Geometry: final body of the model. Coordinates: model frame, mm. A direction names the side the tool comes from. Coordinates: 2 decimals unless noted, no trailing zeros. Loops run counter-clockwise (first coordinate to the right, second up) from the corner with the lowest first, then second, coordinate; pieces in that order, holes last. Notation, with made-up numbers: (-11.75, 31) - (14.25, 31) arc R7 cw to (14.25, 36) - close; hole circle Ø11 at (-34.5, 88). An arc over 180 degrees is marked (long way). Answer in a Markdown table with one row per item.
from build123d import *

# Parameters (mm, degrees)
SKETCH1_W           = 76.2
SKETCH1_H           = 180.975
BOSS_EXTRUDE1_DEPTH = 5.08
SKETCH3_W           = 17.4625
SKETCH3_H           = 9.525
CUT_EXTRUDE1_DEPTH  = 6.08
SKETCH4_W           = 7.62
SKETCH4_H           = 4.826
CUT_EXTRUDE2_DEPTH  = 6.08


with BuildPart() as part:
    # Sketch1 → Boss-Extrude1 (new body)
    with BuildSketch(Plane.XY):
        Rectangle(SKETCH1_W, SKETCH1_H)
    extrude(amount=BOSS_EXTRUDE1_DEPTH)

    # Sketch3 → Cut-Extrude1 (cut, through all)
    with BuildSketch(Plane.XY.offset(5.08)):
        with Locations((0, -85.725)):
            Rectangle(SKETCH3_W, SKETCH3_H)
        with Locations((0, 85.725)):
            Rectangle(SKETCH3_W, SKETCH3_H)
    extrude(amount=-CUT_EXTRUDE1_DEPTH, mode=Mode.SUBTRACT)

    # Sketch4 → Cut-Extrude2 (cut, through all)
    with BuildSketch(Plane.XY.offset(5.08)):
        with Locations((-34.29, 40.513)):
            Rectangle(SKETCH4_W, SKETCH4_H)
        with Locations((34.29, 40.513)):
            Rectangle(SKETCH4_W, SKETCH4_H)
        with Locations((34.29, -40.513)):
            Rectangle(SKETCH4_W, SKETCH4_H)
        with Locations((-34.29, -40.513)):
            Rectangle(SKETCH4_W, SKETCH4_H)
    extrude(amount=-CUT_EXTRUDE2_DEPTH, mode=Mode.SUBTRACT)


solid = part.part
(1) Cut plane A-A on z = 0.8. Output: boundary loops of the cut face in (x, y), then the cut area to 3 significant figures.
Verdict:
| item | result |
|---|---|
| outline | (-38.1, -90.49) - (-8.73, -90.49) - (-8.73, -80.96) - (8.73, -80.96) - (8.73, -90.49) - (38.1, -90.49) - (38.1, -42.93) - (30.48, -42.93) - (30.48, -38.1) - (38.1, -38.1) - (38.1, 38.1) - (30.48, 38.1) - (30.48, 42.93) - (38.1, 42.93) - (38.1, 90.49) - (8.73, 90.49) - (8.73, 80.96) - (-8.73, 80.96) - (-8.73, 90.49) - (-38.1, 90.49) - (-38.1, 42.93) - (-30.48, 42.93) - (-30.48, 38.1) - (-38.1, 38.1) - (-38.1, -38.1) - (-30.48, -38.1) - (-30.48, -42.93) - (-38.1, -42.93) - close |
| area | 13,300 mm² |
(2) Pull-direction query (X, two-part tool) for faces 1 (the face through (8.731, -86, 3)), 2 (the face through (-8.731, 86, 3)), 3 (the face through (-30.48, 40, 3)), 4 (the face through (30.48, 40, 3)); classes: pulls with the +X half, pulls with the -X half, needs draft (parallel to the pull), parting line crosses it, or undercut.
Verdict:
| item | result |
|---|---|
| face 1 | undercut |
| face 2 | undercut |
| face 3 | pulls with the -X half |
| face 4 | pulls with the +X half |
(3) Access query for faces 5 (the face through (-34, 42.926, 3)), 6 (the face through (23, 90.488, 3)), 7 (the face through (34, -38.1, 3)). Directions: +Z, -Z, +X, -X, +Y, -Y. A direction counts if a zero-diameter tool reaches every point of the face in a straight line with its end or side. Return the directions, or none.
Verdict:
| item | result |
|---|---|
| face 5 | +Z, -Z, -X |
| face 6 | +Z, -Z, +X, -X, +Y |
| face 7 | +Z, -Z, +X |
(4) Cut plane B-B on x = 4. Output: boundary loops of the cut face in (y, z).
Verdict:
| item | result |
|---|---|
| outline | (-80.96, 0) - (80.96, 0) - (80.96, 5.08) - (-80.96, 5.08) - close |
(5) First-contact query: pin 1 Ø2.5 at (y, z) = (-41.5, 2) entering from -X; pin 2 Ø1.5 at (x, y) = (21, 0) entering from -Z; pin 3 Ø1.5 at (x, z) = (0, 2.5) entering from -Y. Flat tips, straight axial feed; report the tip coordinate or a pass-through.
Verdict:
| item | result |
|---|---|
| pin 1 | stops at x = -30.48 |
| pin 2 | stops at z = 0 |
| pin 3 | stops at y = -80.96 |
(6) Ray query, probe 1 along Y at (x, z) = (32.5, 3.35); probe 2 along X at (y, z) = (83.5, 0.9); probe 3 along Y at (x, z) = (-3, 3.9). Return the intervals inside material, ascending.
Verdict:
| item | result |
|---|---|
| probe 1 | y = -90.49 to -42.93, -38.1 to 38.1, 42.93 to 90.49 |
| probe 2 | x = -38.1 to -8.73, 8.73 to 38.1 |
| probe 3 | y = -80.96 to 80.96 |
